Work out the finished part from the listing and answer in its coordinate system (mm). Give positions to 0.01 mm unless a question says otherwise; leave off trailing zeros. Order: outer loops, then holes, each group sorted by start corner. A loop starts at its lowest first (then second) coordinate and runs counter-clockwise, first axis right, second up.
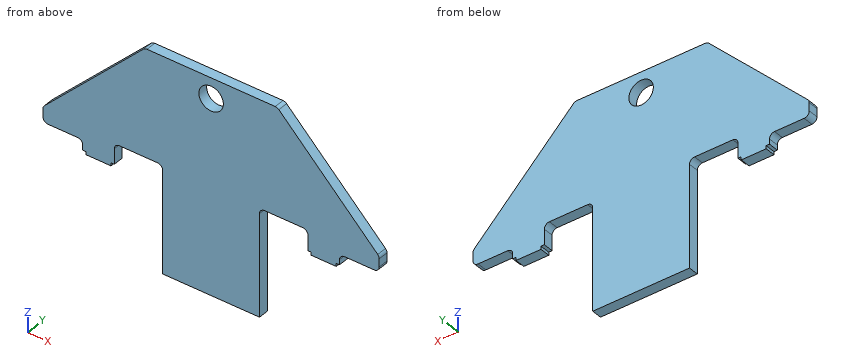
```python
from build123d import *

# Parameters (mm, degrees)
SKETCH1_R               = 12
EXTRUDE1_DEPTH          = 10
FILLET1_R               = 5
ESQUISSE1_W             = 95
ESQUISSE1_H             = 80
ENL_V_MAT_EXTRU_1_DEPTH = 220.886334273


with BuildPart() as part:
    # Sketch1 → Extrude1 (new body)
    with BuildSketch(Plane(origin=(0, 0, 0), x_dir=(1, 0, 0), z_dir=(0, 1, 0))):
        Polygon((-165, -30), (-165, -45), (-65, -145), (65, -145), (165, -45), (165, -30), (126, -30), (126, -20), (122.75, -20), (122.75, -17), (98.25, -17), (98.25, -20), (95, -20), (95, -40), (47.5, -40), (47.5, 123.333333333), (15, 145), (-15, 145), (-47.5, 123.333333333), (-47.5, -40), (-95, -40), (-95, -20), (-98.25, -20), (-98.25, -17), (-122.75, -17), (-122.75, -20), (-126, -20), (-126, -30), align=None)
        with Locations(Location((0, 113, 0), (0, 0, 270))):
            Circle(SKETCH1_R, mode=Mode.SUBTRACT)
        with Locations(Location((0, -125, 0), (0, 0, 270))):
            Circle(SKETCH1_R, mode=Mode.SUBTRACT)
    extrude(amount=EXTRUDE1_DEPTH)

    # Fillet1
    fillet1_edges = [part.edges().sort_by_distance(p)[0] for p in [
        (-126, 5, 30),
        (-95, 5, 40),
        (-47.5, 5, 40),
        (-47.5, 5, -123.333333333),
        (-15, 5, -145),
        (15, 5, -145),
        (47.5, 5, -123.333333333),
        (47.5, 5, 40),
        (95, 5, 40),
        (126, 5, 30),
        (165, 5, 30),
        (165, 5, 45),
        (65, 5, 145),
        (-65, 5, 145),
        (-165, 5, 45),
        (-165, 5, 30),
    ]]
    fillet(fillet1_edges, radius=FILLET1_R)

    # Esquisse1 → Enlèv. mat.-Extru.1 (cut, through all)
    with BuildSketch(Plane(origin=(0, 10, 0), x_dir=(1, 0, 0), z_dir=(0, 1, 0))):
        with Locations((0, 105)):
            Rectangle(ESQUISSE1_W, ESQUISSE1_H)
    extrude(amount=-ENL_V_MAT_EXTRU_1_DEPTH, mode=Mode.SUBTRACT)


solid = part.part
```
1. Given P1, Ø3.5, axis at y = 3.5, z = 18.5, coming from the +X side; P2, Ø5, axis at x = -107.5, y = 7, coming from the -Z side; P3, Ø1, axis at y = 4.5, z = 108.5, coming from the +X side, each flat-ended and moving along its own axis, determine where each tip first touches the part or whether it passes through.
Findings below:
P1: stops at x = 126
P2: stops at z = 17
P3: stops at x = 102
2. The part is cut by section A-A (z = 125). Write down the section's boundary in (x, y).
Findings below:
outline: (-85, 0) - (-12, 0) - (-12, 10) - (-85, 10) - close; (12, 0) - (85, 0) - (85, 10) - (12, 10) - close
3. The part is cut by section C-C (x = -113). Write down the section's boundary in (y, z).
Findings below:
outline: (0, 17) - (10, 17) - (10, 97) - (0, 97) - close
4. The part is cut by section D-D (z = 76). Write down the section's boundary in (x, y), then the cut area to 3 significant figures.
Findings below:
outline: (-134, 0) - (134, 0) - (134, 10) - (-134, 10) - close
area: 2,680 mm2
5. Straight lines are drawn through the part: probe 1 along X at (y, z) = (9.75, 39); probe 2 along X at (y, z) = (4, 4.5); probe 3 along Z at (x, y) = (-115, 9.5). For each, find the intervals that lie inside material, in ascending order.
Findings below:
probe 1: x = -165 to -93, -49.5 to 49.5, 93 to 165
probe 2: x = -47.5 to 47.5
probe 3: z = 17 to 95
6. The part is cut by section B-B (x = 0). Write down the section's boundary in (y, z).
Findings below:
outline: (0, -65) - (10, -65) - (10, 113) - (0, 113) - close; (0, 137) - (10, 137) - (10, 145) - (0, 145) - close
